For this review, take the finished solid that the model builds, in its own axes (mm). Face numbers are marked on the shaded views. A direction names the side the tool comes from. Round coordinates to 2 decimals unless told otherwise and drop trailing zeros. Loops run counter-clockwise (first coordinate to the right, second up) from the corner with the lowest first, then second, coordinate; pieces in that order, holes last. Notation, with made-up numbers: (78, 69) -> (112, 69) arc R9 ccw to (112, 75) -> close; hole circle Ø4 at (-36, 85). An arc over 180 degrees is marked (long way). Use one line per item in the form item = value. Start each with the question number.
from build123d import *

# Parameters (mm, degrees)
F1_DEPTH      = 6.35
F2_W          = 3.175
F2_H          = 6.35
F4_ANGLE_BACK = 22.5
F4_ANGLE      = 45
F5_W          = 6.35
F5_H          = 12.7
F5_W_2        = 13.0048
F6_DEPTH      = 12.7


with BuildPart() as f1:
    # F0 (on Top) → F1 (new body)
    with BuildSketch(Plane.XY):
        with BuildLine():
            Line((30.5767274074, 73.81875), (40.3994116005, 97.5328073978))
            ThreePointArc((40.3994116005, 97.5328073978), (0, 105.56875), (-40.3994116005, 97.5328073978))
            Line((-40.3994116005, 97.5328073978), (-30.5767274074, 73.81875))
            Line((-30.5767274074, 73.81875), (30.5767274074, 73.81875))
        make_face()
    extrude(amount=F1_DEPTH)

    # F2 (on Right) → F4 (revolve)
    with BuildSketch(Plane.YZ, mode=Mode.PRIVATE) as f4_sk:
        with Locations((103.98125, -3.175)):
            Rectangle(F2_W, F2_H)
    revolve(f4_sk.sketch.rotate(Axis((0, 0, 6.6674984992), (0, 0, -1)), -F4_ANGLE_BACK), axis=Axis((0, 0, 6.6674984992), (0, 0, -1)), revolution_arc=F4_ANGLE)

    # F5 (on face) → F6 (cut, symmetric)
    with BuildSketch(Plane(origin=(0, 0, 0), x_dir=(1, 0, 0), z_dir=(0, 0, -1))):
        with Locations((0, -80.16875)):
            Rectangle(F5_W, F5_H)
        with Locations((0, -105.56875)):
            Rectangle(F5_W_2, F5_H)
    extrude(amount=F6_DEPTH, both=True, mode=Mode.SUBTRACT)


solid = f1.part
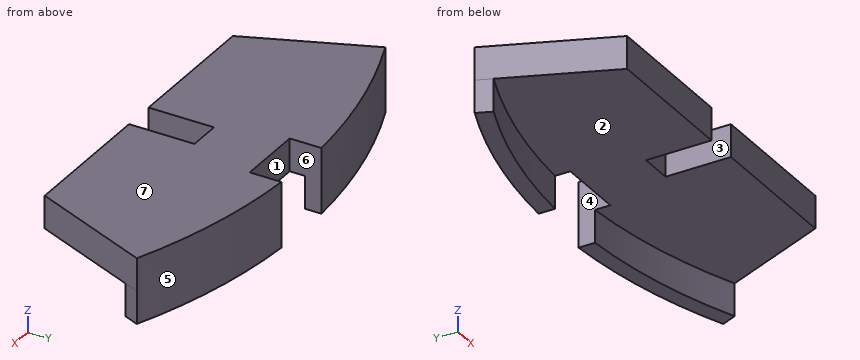
Item 1: Take a section at B-B on y = 85. Give the boundary of the cut face in (x, z) (3 decimals), plus the area to 3 significant figures.
Item 2: Take a section at D-D on x = -14.5. Give the boundary of the cut face in (y, z).
Item 3: Draft analysis for pull direction X (two halves, no side actions). For the marked faces 4, 5, 6 and 7, state which applies: +X half, -X half, draft (parallel to the pull), parting line (faces both ways), or undercut.
Item 4: Take a section at C-C on z = 5.5. Give the boundary of the cut face in (x, y) (1 decimal), plus the area to 3 significant figures.
Item 5: For P1, Ø5, axis at y = 82, z = 2, coming from the -X side; P2, Ø3, axis at x = 0.5, z = 3, coming from the -Y side; P3, Ø3, axis at y = 80.5, z = 2, coming from the +X side; P4, Ø4, axis at x = 5, z = -3, coming from the +Y side, all flat-tipped, find the tip position at first contact; note any pin that passes through.
Item 6: Take a section at A-A on z = -2. Give the boundary of the cut face in (x, y), plus the area to 3 significant figures.
Item 7: Machinability: for the marked faces 1, 2 and 3, which of the approach directions +Z, -Z, +X, -X, +Y, -Y give a long, thin tool a straight path to every point of the face, cutting with its end or side? Answer none if there is none.
Item 8: Wall thickness on line 1 (Y direction, x = -2, z = 2.5); line 2 (Z direction, x = -27.5, y = 77.5); line 3 (X direction, y = 78, z = 1.25) (3 decimals): over which ranges is each line inside the solid? List them lowest first.
Results:
q1.outline = (-35.208, 0) -> (-3.175, 0) -> (-3.175, 6.35) -> (-35.208, 6.35) -> close; (3.175, 0) -> (35.208, 0) -> (35.208, 6.35) -> (3.175, 6.35) -> close
q1.area = 407 mm2
q2.outline = (73.82, 0) -> (101.36, 0) -> (101.36, -6.35) -> (104.57, -6.35) -> (104.57, 6.35) -> (73.82, 6.35) -> close
q3.face_4 = undercut
q3.face_5 = +X half
q3.face_6 = undercut
q3.face_7 = draft
q4.outline = (-40.4, 97.5) -> (-30.6, 73.8) -> (-3.2, 73.8) -> (-3.2, 86.5) -> (3.2, 86.5) -> (3.2, 73.8) -> (30.6, 73.8) -> (40.4, 97.5) arc R105.6 ccw to (6.5, 105.4) -> (6.5, 99.2) -> (-6.5, 99.2) -> (-6.5, 105.4) arc R105.6 ccw to start
q4.area = 1,960 mm2
q5.P1 = -35
q5.P2 = 86.52
q5.P3 = 33.97
q5.P4 = 105.37
q6.outline = (-40.4, 97.53) -> (-39.18, 94.6) arc R102.39 cw to (-6.5, 102.19) -> (-6.5, 105.37) arc R105.57 ccw to start; (6.5, 102.19) arc R102.39 cw to (39.18, 94.6) -> (40.4, 97.53) arc R105.57 ccw to (6.5, 105.37) -> close
q6.area = 218 mm2
q7.face_1 = +Z, -Z, +Y
q7.face_2 = -Z, -Y
q7.face_3 = +Z, -Z, -Y
q8.line_1 = 86.52 to 99.22
q8.line_2 = 0 to 6.35
q8.line_3 = -32.309 to -3.175, 3.175 to 32.309
